from build123d import *

# Parameters (mm, degrees)
SZKIC1_W                       = 45
SZKIC1_H                       = 40
ODGI_CIE_BAZOWE1_DEPTH         = 2
ODGI_CIE_START                 = -22.5
ODGI_CIE_KRAW_DZI1_DEPTH       = 45
ODGI_CIE_KRAW_DZI1_2_OUTLINE_W = 31
ODGI_CIE_KRAW_DZI1_2_OUTLINE_H = 2
ODGI_CIE_KRAW_DZI1_2_DEPTH     = 45
WYTNIJ_WYCI_GNI_CIE1_REACH     = 45.212
SZKIC13_R                      = 4.5
WYTNIJ_WYCI_GNI_CIE2_DEPTH     = 56.38275905
WYTNIJ_WYCI_GNI_CIE3_REACH     = 57.383
SZKIC14_R                      = 2


# Read off the part's stored shape, not the designer's step: Odgięcie krawędzi1
# Sheet-metal steps are written as plain solids
with BuildPart() as part:
    # Szkic1 → Odgięcie bazowe1 (new body)
    with BuildSketch(Plane(origin=(0, 0, 0), x_dir=(1, 0, 0), z_dir=(0, 1, 0))):
        Rectangle(SZKIC1_W, SZKIC1_H)
    extrude(amount=-ODGI_CIE_BAZOWE1_DEPTH)

    # Odgięcie krawędzi1 outline → Odgięcie krawędzi1 (cut)
    with BuildSketch(Plane.YZ.offset(ODGI_CIE_START)):
        with BuildLine():
            ThreePointArc((0, -20), (-1.414213562, -19.414213562), (-2, -18))
            Line((-2, -18), (-2, -20))
            Line((-2, -20), (0, -20))
        make_face()
        with BuildLine():
            Line((-2, 20), (-2, 18))
            ThreePointArc((-2, 18), (-1.414213562, 19.414213562), (0, 20))
            Line((0, 20), (-2, 20))
        make_face()
    extrude(amount=ODGI_CIE_KRAW_DZI1_DEPTH, mode=Mode.SUBTRACT)

    # Odgi_cie kraw_dzi1 2 outline → Odgi_cie kraw_dzi1 2 (add)
    with BuildSketch(Plane.YZ.offset(ODGI_CIE_START)):
        with Locations((15.5, -19)):
            Rectangle(ODGI_CIE_KRAW_DZI1_2_OUTLINE_W, ODGI_CIE_KRAW_DZI1_2_OUTLINE_H)
        with Locations((15.5, 19)):
            Rectangle(ODGI_CIE_KRAW_DZI1_2_OUTLINE_W, ODGI_CIE_KRAW_DZI1_2_OUTLINE_H)
    extrude(amount=ODGI_CIE_KRAW_DZI1_2_DEPTH)

    # Szkic12 → Wytnij-wyciągnięcie1 (cut, up to next)
    with BuildSketch(Plane(origin=(0, 0, 0), x_dir=(1, 0, 0), z_dir=(0, 1, 0)), mode=Mode.PRIVATE) as wytnij_wyci_gni_cie1_sk1:
        with BuildLine():
            Line((-9.5, -13), (-9.5, 13))
            ThreePointArc((-9.5, 13), (-8, 14.5), (-6.5, 13))
            Line((-6.5, 13), (-6.5, -13))
            ThreePointArc((-6.5, -13), (-8, -14.5), (-9.5, -13))
        make_face()
    wytnij_wyci_gni_cie1_tool1 = extrude(wytnij_wyci_gni_cie1_sk1.sketch, amount=-WYTNIJ_WYCI_GNI_CIE1_REACH, mode=Mode.PRIVATE) & part.part
    wytnij_wyci_gni_cie1 = wytnij_wyci_gni_cie1_tool1.solids().sort_by_distance((-8, 0, 0))[0]
    add(wytnij_wyci_gni_cie1, mode=Mode.SUBTRACT)

    # Lustro1: Wytnij-wyciągnięcie1 across plane
    add(wytnij_wyci_gni_cie1.mirror(Plane(origin=(0, 0, 0), x_dir=(0, 0, 1), z_dir=(1, 0, 0))), mode=Mode.SUBTRACT)

    # Szkic13 → Wytnij-wyciągnięcie2 (cut, through all)
    with BuildSketch(Plane(origin=(0, 0, -20), x_dir=(-1, 0, 0), z_dir=(0, 0, -1))):
        with Locations(Location((0, 21, 0), (0, 0, 90))):
            Circle(SZKIC13_R)
    extrude(amount=-WYTNIJ_WYCI_GNI_CIE2_DEPTH, mode=Mode.SUBTRACT)

    # Szkic14 → Wytnij-wyciągnięcie3 (cut, up to next)
    with BuildSketch(Plane(origin=(0, 0, -20), x_dir=(-1, 0, 0), z_dir=(0, 0, -1)), mode=Mode.PRIVATE) as wytnij_wyci_gni_cie3_sk1:
        with Locations(Location((-17.5, 13, 0), (0, 0, 90))):
            Circle(SZKIC14_R)
    wytnij_wyci_gni_cie3_tool1 = extrude(wytnij_wyci_gni_cie3_sk1.sketch, amount=-WYTNIJ_WYCI_GNI_CIE3_REACH, mode=Mode.PRIVATE) & part.part
    # Szkic14 → Wytnij-wyciągnięcie3 (cut, up to next)
    with BuildSketch(Plane(origin=(0, 0, -20), x_dir=(-1, 0, 0), z_dir=(0, 0, -1)), mode=Mode.PRIVATE) as wytnij_wyci_gni_cie3_sk2:
        with Locations(Location((17.5, 13, 0), (0, 0, 90))):
            Circle(SZKIC14_R)
    wytnij_wyci_gni_cie3_tool2 = extrude(wytnij_wyci_gni_cie3_sk2.sketch, amount=-WYTNIJ_WYCI_GNI_CIE3_REACH, mode=Mode.PRIVATE) & part.part
    add(wytnij_wyci_gni_cie3_tool1.solids().sort_by_distance((17.5, 13, -20))[0], mode=Mode.SUBTRACT)
    add(wytnij_wyci_gni_cie3_tool2.solids().sort_by_distance((-17.5, 13, -20))[0], mode=Mode.SUBTRACT)


solid = part.part
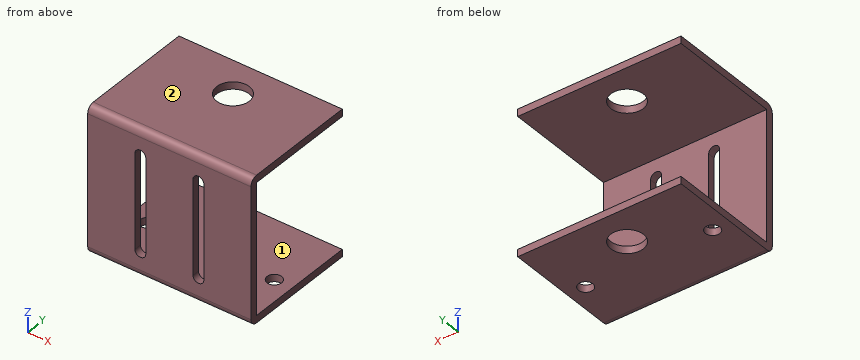
Geometry check sheet. Reference: the model listing, model coordinates, mm. Face numbers are marked on the shaded views. A direction names the side the tool comes from. Round coordinates to 2 decimals unless told otherwise and drop trailing zeros. Write each loop counter-clockwise with the first axis right and the second up, starting at its lowest first coordinate (ties: lowest second). Pieces come first, ordered by that corner, then holes. Notation, with made-up numbers: (1, 55.5) -> (25, 55.5) arc R12 cw to (25, 67.5) -> close; hole circle Ø8 at (25, -17.75). An arc over 180 degrees is marked (long way). One line per item, written item: value. Start each with the question number.
(1) Go/stop test with a flat-tipped pin: pin 1 Ø1.5 at (x, z) = (-3.5, -10.5) entering from +Y. Record where the tip stops, or that it passes through.
(2) Cross-section at C-C, the plane y = 21. Record the cut outline in (x, z).
(3) Cross-section at B-B, the plane z = 5.5. Record the cut outline in (x, y), and give its area (3 significant figures).
(4) Cross-section at A-A, the plane x = -8. Record the cut outline in (y, z), and give its area (3 significant figures).
(5) Scan lines: line 1 (Z direction, x = 3, y = 13.5); line 2 (X direction, y = 13, z = -18.7); line 3 (X direction, y = 21, z = -19.5). Record each from-to range of solid material in increasing order. Write a range as [from, to].
(6) Cross-section at D-D, the plane y = 6.5. Record the cut outline in (x, z).
(7) Access from +Z, -Z, +X, -X, +Y, -Y to the whole of each face (thin tool, end or side, straight path). Record for the marked faces 1 and 2.
Answer:
1. pin 1: y = 0
2. outline: (-22.5, -20) -> (-4.5, -20) -> (-4.5, -18) -> (-22.5, -18) -> close; (-22.5, 18) -> (-4.5, 18) -> (-4.5, 20) -> (-22.5, 20) -> close; (4.5, -20) -> (22.5, -20) -> (22.5, -18) -> (4.5, -18) -> close; (4.5, 18) -> (22.5, 18) -> (22.5, 20) -> (4.5, 20) -> close
3. outline: (-22.5, -2) -> (-9.5, -2) -> (-9.5, 0) -> (-22.5, 0) -> close; (-6.5, -2) -> (6.5, -2) -> (6.5, 0) -> (-6.5, 0) -> close; (9.5, -2) -> (22.5, -2) -> (22.5, 0) -> (9.5, 0) -> close
3. area: 78.0 mm²
4. outline: (-2, -18) arc R2 ccw to (0, -20) -> (31, -20) -> (31, -18) -> (0, -18) -> (0, -14.5) -> (-2, -14.5) -> close; (-2, 14.5) -> (0, 14.5) -> (0, 18) -> (31, 18) -> (31, 20) -> (0, 20) arc R2 ccw to (-2, 18) -> close
4. area: 144 mm²
5. line 1: [-20, -18], [18, 20]
5. line 2: [-22.5, -19.5], [-15.5, 15.5], [19.5, 22.5]
5. line 3: [-22.5, -4.5], [4.5, 22.5]
6. outline: (-22.5, -20) -> (22.5, -20) -> (22.5, -18) -> (-22.5, -18) -> close; (-22.5, 18) -> (22.5, 18) -> (22.5, 20) -> (-22.5, 20) -> close
7. face 1: +X, -X, +Y
7. face 2: +Z, +X, -X, +Y, -Y
